Drawing for the job (mm, zero at the part's lowest x, y, z). A direction names the side the tool comes from. Give positions to 0.01 mm unless a question says otherwise; leave off trailing zeros. Loops run counter-clockwise (first coordinate to the right, second up) from the corner with the lowest first, then second, coordinate; pieces in that order, holes last.
1) Wall check: line 1 (Y direction, x = 3.15, z = 64); line 2 (Z direction, x = 1.25, y = 26); line 3 (Z direction, x = 4.5, y = 45). Give the ranges that are in metal, low to high.
2) Band-saw the part on A-A on z = 64. List the corners of the cut face in (x, y).
3) 3-axis set-ups, long thin cutter, end or side, ignore diameter. For the marked faces 1, 2 and 3: which of +Z, -Z, +X, -X, +Y, -Y reach the whole face in a straight line?
4) Two-plate mould, pull along Z, no slides. Class the marked faces 4, 5 and 6: +Z half, -Z half, draft (parallel to the pull), parting line (faces both ways), or undercut.
5) Flat gauge pins, fed straight in: P1, Ø10, axis at y = 28, z = 44.5, coming from the +X side; P2, Ø5.5, axis at y = 27, z = 64, coming from the +X side; P3, Ø1.5, axis at x = 1.5, y = 38, coming from the +Z side; P4, Ø23, axis at y = 8, z = 20.5, coming from the -X side. Where does each tip first touch, or does it go through?
6) Band-saw the part on D-D on z = 40.5. List the corners of the cut face in (x, y), then the cut area to 3 significant figures.
7) Band-saw the part on B-B on x = 7. List the corners of the cut face in (y, z), then the cut area to 3 significant figures.
8) Band-saw the part on C-C on y = 27. List the corners of the cut face in (x, z).
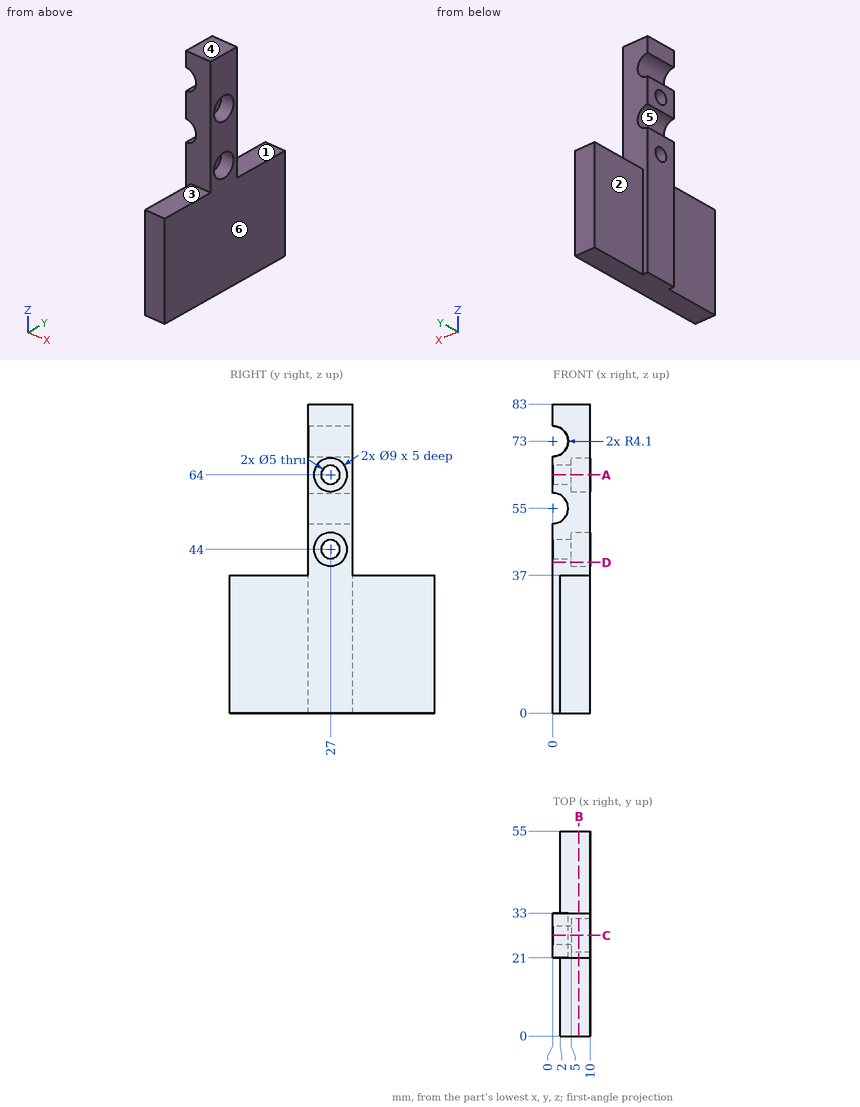
Findings below:
1. line 1: y = 21 to 24.5, 29.5 to 33
1. line 2: z = 0 to 41.71, 46.29 to 51.1, 58.9 to 61.71, 66.29 to 69.1, 76.9 to 83
1. line 3: z = 0 to 37
2. outline: (0, 21) - (10, 21) - (10, 22.5) - (5, 22.5) - (5, 24.5) - (0, 24.5) - close; (0, 29.5) - (5, 29.5) - (5, 31.5) - (10, 31.5) - (10, 33) - (0, 33) - close
3. face 1: +Z, +X, -X, +Y
3. face 2: +Z, -Z, -X, +Y
3. face 3: +Z, +X, -X, -Y
4. face 4: +Z half
4. face 5: undercut
4. face 6: draft
5. P1: stops at x = 10
5. P2: stops at x = 5
5. P3: stops at z = 37
5. P4: stops at x = 2
6. outline: (0, 21) - (10, 21) - (10, 24.17) - (5, 24.17) - (5, 29.83) - (10, 29.83) - (10, 33) - (0, 33) - close
6. area: 91.7 mm2
7. outline: (0, 0) - (55, 0) - (55, 37) - (33, 37) - (33, 83) - (21, 83) - (21, 37) - (0, 37) - close; hole circle Ø9 at (27, 44); hole circle Ø9 at (27, 64)
7. area: 2,460 mm2
8. outline: (0, 0) - (10, 0) - (10, 39.5) - (5, 39.5) - (5, 41.5) - (0, 41.5) - close; (0, 46.5) - (5, 46.5) - (5, 48.5) - (10, 48.5) - (10, 59.5) - (5, 59.5) - (5, 61.5) - (0, 61.5) - (0, 59.1) arc R4.1 cw to (0, 50.9) - close; (0, 66.5) - (5, 66.5) - (5, 68.5) - (10, 68.5) - (10, 83) - (0, 83) - (0, 77.1) arc R4.1 cw to (0, 68.9) - close
